Read the model definition and answer for the solid it produces. Units are mm, in the model's axes. Face numbers are marked on the shaded views. A direction names the side the tool comes from. Give positions to 0.01 mm unless a question says otherwise; leave off trailing zeros. Loops run counter-clockwise (first coordinate to the right, second up) from the corner with the lowest first, then second, coordinate; pieces in that order, holes last. Notation, with made-up numbers: (10.25, 48.25) -> (42.25, 48.25) arc R20 cw to (42.25, 62.25) -> close; hole circle Ø1 at (-26, 53.5). An arc over 180 degrees is marked (long way). Answer as CSV lines item,"result". Start each with the question number.
```python
from build123d import *

# Parameters (mm, degrees)
SZKIC1_W                             = 55.4
SZKIC1_H                             = 28
ODGI_CIE_BAZOWE1_DEPTH               = 2
OTWORY_USTALAJ_CE_3_0MM1_D           = 3
OTWORY_USTALAJ_CE_3_0MM1_DEPTH       = 17
OTWORY_USTALAJ_CE_3_0MM1_TIP         = 0.901290929
ODGI_CIE_KRAW_DZI1_STRIP_W           = 9.4732
ODGI_CIE_KRAW_DZI1_STRIP_H           = 2
ODGI_CIE_KRAW_DZI1_STRIP_CUT_DEPTH   = 55.4
ODGI_CIE_KRAW_DZI1_STRIP_2_W         = 9.4732
ODGI_CIE_KRAW_DZI1_STRIP_2_H         = 2
ODGI_CIE_KRAW_DZI1_STRIP_CUT_2_DEPTH = 55.4
ODGI_CIE_KRAW_DZI1_DEPTH             = 55.4
ODGI_CIE_KRAW_DZI1_BEND_DEPTH        = 55.4
OTW_R_GWINTOWANY_M3X0_51_D           = 2.5


# Sheet-metal steps are written as plain solids
with BuildPart() as part:
    # Szkic1 → Odgięcie bazowe1 (new body)
    with BuildSketch(Plane.XY):
        Rectangle(SZKIC1_W, SZKIC1_H)
    extrude(amount=-ODGI_CIE_BAZOWE1_DEPTH)

    # Otwory ustalające Ø3.0mm1
    with Locations(Plane(origin=(0, 0, -2), x_dir=(-1, 0, 0), z_dir=(0, 0, -1))):
        with Locations((-10, 10), (10, 10), (10, -10), (-10, -10)):
            Hole(OTWORY_USTALAJ_CE_3_0MM1_D / 2, depth=OTWORY_USTALAJ_CE_3_0MM1_DEPTH)
            with Locations((0, 0, -(OTWORY_USTALAJ_CE_3_0MM1_DEPTH + OTWORY_USTALAJ_CE_3_0MM1_TIP / 2))):  # 118° drill point
                Cone(0, OTWORY_USTALAJ_CE_3_0MM1_D / 2, OTWORY_USTALAJ_CE_3_0MM1_TIP, mode=Mode.SUBTRACT)

    # Odgięcie krawędzi1 strip (across the edge) → Odgięcie krawędzi1 strip cut (cut)
    with BuildSketch(Plane(origin=(27.7, 14, 0), x_dir=(0, -1, 0), z_dir=(-1, 0, 0))):
        with Locations((-4, -1)):
            Rectangle(ODGI_CIE_KRAW_DZI1_STRIP_W, ODGI_CIE_KRAW_DZI1_STRIP_H)
    extrude(amount=ODGI_CIE_KRAW_DZI1_STRIP_CUT_DEPTH, mode=Mode.SUBTRACT)

    # Odgięcie krawędzi1 strip 2 (across the edge) → Odgięcie krawędzi1 strip cut 2 (cut)
    with BuildSketch(Plane(origin=(-27.7, -14, 0), x_dir=(0, 1, 0), z_dir=(1, 0, 0))):
        with Locations((-4, -1)):
            Rectangle(ODGI_CIE_KRAW_DZI1_STRIP_2_W, ODGI_CIE_KRAW_DZI1_STRIP_2_H)
    extrude(amount=ODGI_CIE_KRAW_DZI1_STRIP_CUT_2_DEPTH, mode=Mode.SUBTRACT)

    # Odgięcie krawędzi1 section (across the edge) → Odgięcie krawędzi1 (add)
    with BuildSketch(Plane(origin=(27.7, 14, 0), x_dir=(0, -1, 0), z_dir=(-1, 0, 0))):
        with BuildLine():
            Line((-2, 0.7366), (-2, 43))
            Line((-2, 43), (0, 43))
            Line((0, 43), (0, 0.7366))
            ThreePointArc((0, 0.7366), (0.215745145, 0.215745145), (0.7366, 0))
            Line((0.7366, 0), (0.7366, -2))
            ThreePointArc((0.7366, -2), (-1.198468417, -1.198468417), (-2, 0.7366))
        make_face()
    extrude(amount=ODGI_CIE_KRAW_DZI1_DEPTH)

    # Odgięcie krawędzi1 section 2 (across the edge) → Odgięcie krawędzi1 bend (add)
    with BuildSketch(Plane(origin=(-27.7, -14, 0), x_dir=(0, 1, 0), z_dir=(1, 0, 0))):
        with BuildLine():
            Line((-2, 0.7366), (-2, 43))
            Line((-2, 43), (0, 43))
            Line((0, 43), (0, 0.7366))
            ThreePointArc((0, 0.7366), (0.215745145, 0.215745145), (0.7366, 0))
            Line((0.7366, 0), (0.7366, -2))
            ThreePointArc((0.7366, -2), (-1.198468417, -1.198468417), (-2, 0.7366))
        make_face()
    extrude(amount=ODGI_CIE_KRAW_DZI1_BEND_DEPTH)

    # Otwór gwintowany M3x0.51 (through all)
    with Locations(Plane(origin=(0, 16, 0), x_dir=(1, 0, 0), z_dir=(0, 1, 0))):
        with Locations((-24.7, -35.3), (-24.7, -15.3), (24.7, -35.3), (24.7, -15.3)):
            Hole(OTW_R_GWINTOWANY_M3X0_51_D / 2)


solid = part.part
```
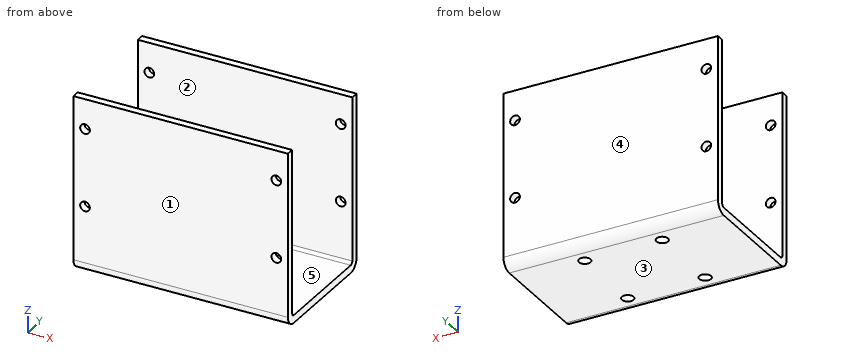
(1) Find section A-A on z = 9. Write down the section's boundary in (x, y), then the cut area to 3 significant figures.
(2) Each of these flat-tipped pins is pushed along its axis until it touches: P1, Ø2, axis at x = -24.7, z = 15.3, coming from the -Y side; P2, Ø10, axis at x = -17, y = -5, coming from the +Z side. Where does it stop, or does it pass through?
(3) Find section B-B on y = -10. Write down the section's boundary in (x, z), then the cut area to 3 significant figures.
(4) The mould has two halves that part along Y. Classify the marked faces 1, 2 and 3: pulls with the +Y half, pulls with the -Y half, needs draft (parallel to the pull), parting line crosses it, or undercut.
(5) Find section D-D on x = 10. Write down the section's boundary in (y, z).
(6) Find the intervals of material crossed by line 1 along X through (y, z) = (-14.5, 15.3); line 2 along Y through (x, z) = (-5, 20); line 3 along Z through (x, y) = (-24.7, 14.6), in increasing order. Write a range as from..to.
(7) A tool of negligible diameter and unlimited length cuts with its end or side. For the marked faces 4 and 5, from which of +Z, -Z, +X, -X, +Y, -Y can it reach the whole face along a straight path? Write none if from no direction.
(8) Find section C-C on x = 17. Write down the section's boundary in (y, z).
Answer block:
1,outline,"(-27.7, -16) -> (27.7, -16) -> (27.7, -14) -> (-27.7, -14) -> close; (-27.7, 14) -> (27.7, 14) -> (27.7, 16) -> (-27.7, 16) -> close"
1,area,"222 mm2"
2,P1,"passes through"
2,P2,"stops at z = 0"
3,outline,"(-27.7, -2) -> (-11.5, -2) -> (-11.5, 0) -> (-27.7, 0) -> close; (-8.5, -2) -> (8.5, -2) -> (8.5, 0) -> (-8.5, 0) -> close; (11.5, -2) -> (27.7, -2) -> (27.7, 0) -> (11.5, 0) -> close"
3,area,"98.8 mm2"
4,face 1,"pulls with the -Y half"
4,face 2,"undercut"
4,face 3,"needs draft"
5,outline,"(-16, 0.74) arc R2.74 ccw to (-13.26, -2) -> (-11.5, -2) -> (-11.5, 0) -> (-13.26, 0) arc R0.74 cw to (-14, 0.74) -> (-14, 43) -> (-16, 43) -> close; (-8.5, -2) -> (8.5, -2) -> (8.5, 0) -> (-8.5, 0) -> close; (11.5, -2) -> (13.26, -2) arc R2.74 ccw to (16, 0.74) -> (16, 43) -> (14, 43) -> (14, 0.74) arc R0.74 cw to (13.26, 0) -> (11.5, 0) -> close"
6,line 1,"x = -27.7..-25.95, -23.45..23.45, 25.95..27.7"
6,line 2,"y = -16..-14, 14..16"
6,line 3,"z = -1.65..14.05, 16.55..34.05, 36.55..43"
7,face 4,"+Z, -Z, +X, -X, +Y"
7,face 5,"+Z, +X, -X"
8,outline,"(-16, 0.74) arc R2.74 ccw to (-13.26, -2) -> (13.26, -2) arc R2.74 ccw to (16, 0.74) -> (16, 43) -> (14, 43) -> (14, 0.74) arc R0.74 cw to (13.26, 0) -> (-13.26, 0) arc R0.74 cw to (-14, 0.74) -> (-14, 43) -> (-16, 43) -> close"
